Source: CAD feature listing. Evaluate the final solid. Frame: model axes, mm. A direction names the side the tool comes from. Coordinates: 2 decimals unless noted, no trailing zeros. Order: outer loops, then holes, each group sorted by start corner. A loop starts at its lowest first (then second) coordinate and runs counter-clockwise, first axis right, second up.
Autodesk Inventor part; units mm, degrees
ref_plane "YZ Plane" through (0, 0, 0) normal (1, 0, 0) x (0, 1, 0)
ref_plane "XZ Plane" through (0, 0, 0) normal (0, 1, 0) x (-1, 0, 0)
ref_plane "XY Plane" through (0, 0, 0) normal (0, 0, 1) x (1, 0, 0)
sketch "Sketch1" plane through (0, 0, 0) normal (0, 0, 1) x (1, 0, 0)
  line L0 (0, 0) -> (-50.8, 0)
  line L1 (-50.8, 0) -> (-50.8, -12.7)
  line L2 (-50.8, -12.7) -> (-38.1, -12.7)
  line L3 (-12.0663, -25.4) -> (-12.0663, -48.26)
  line L4 (-5, -48.26) -> (-5, -16.764)
  line L5 (-5, -16.764) -> (0, -16.764)
  line L6 (0, -16.764) -> (0, 0)
  line L7 (-12.0663, -48.26) -> (-5, -48.26)
  line L8 (-38.1, -12.7) -> (-38.1, -25.4)
  line L9 (-38.1, -25.4) -> (-12.0663, -25.4)
  dimension "d0" = 50.8
  dimension "d1" = 5
  dimension "d2" = 12.0663
  dimension "d13" = 35.56
  dimension "d15" = 31.496
  dimension "d38" = 12.7
  dimension "d39" = 38.1
revolve "Revolution1" add sketch "Sketch1" angle 360 about axis through (0, -16.764, 0) along (0, 1, 0)
sketch "Sketch5" plane through (0, 0, 0) normal (0, 1, 0) x (1, 0, 0)
  circle A0 centre (0, 0) radius 5
  line L0 (9.815, 0) -> (4.9075, -8.5)
  line L1 (4.9075, -8.5) -> (-4.9075, -8.5)
  line L2 (-4.9075, -8.5) -> (-9.815, 0)
  line L3 (-9.815, 0) -> (-4.9075, 8.5)
  line L4 (-4.9075, 8.5) -> (4.9075, 8.5)
  line L5 (4.9075, 8.5) -> (9.815, 0)
  point P0 (0, 0)
  point P1 (0, 0)
  dimension "d16" = 17
extrude "Extrusion1" cut sketch "Sketch5" against normal blind 12.7 contours A0 | L0 L1 L2 L3 L4 L5
sketch "Sketch7" plane through (0, -12.7, 0) normal (0, -1, 0) x (1, 0, 0)
  circle A0 centre (0, 0) radius 50.8
  line L0 (47.0929, -19.05) -> (85.1929, -19.05)
  line L1 (85.1929, -19.05) -> (85.1929, -31.75)
  line L2 (85.1929, -31.75) -> (39.6557, -31.75)
  circle A1 centre (0, 0) radius 5 construction
  line L3 (0, 0) -> (5, 0) construction
  line L4 (50.8, 0) -> (83.823, 0) construction
  dimension "d23" = 38.1
  dimension "d24" = 12.7
  dimension "d25" = 19.05
extrude "Extrusion3" add sketch "Sketch7" against normal blind 12.7 contours A0 L0 L1 L2
sketch "Sketch8" plane through (39.6557, 0, -31.75) normal (0, 1, 0) x (1, 0, 0)
  line L0 (45.5371, -12.7) -> (45.5371, 0)
  line L1 (45.5371, 0) -> (0, 0)
  line L2 (7.4371, -12.7) -> (45.5371, -12.7)
  line L3 (35.8511, -107.95) -> (35.8511, 44.45)
  line L4 (26.3261, -107.95) -> (26.3261, 44.45)
  line L5 (45.5371, -12.7) -> (23.3121, -12.7)
  line L6 (23.3121, -12.7) -> (23.3121, 0)
  line L7 (23.3121, 0) -> (45.5371, 0)
  line L8 (45.5371, 0) -> (45.5371, -12.7)
  point P0 (-39.6557, -31.75)
  point P1 (23.3121, 0)
  point P2 (23.3121, -12.7)
  dimension "d28" = 22.225
extrude "Extrusion4" add sketch "Sketch8" along normal blind 19.05
sketch "Sketch9" plane through (85.1929, -12.7, -31.75) normal (0, 0, -1) x (-1, 0, 0)
  line L0 (22.225, 12.7) -> (22.225, 31.75)
  line L1 (0, 31.75) -> (22.225, 31.75)
  arc A0 (16.0423, 14.3621) -> (12.8546, 14.3621) centre (14.4485, 18.85) ccw
  line L2 (0, 0) -> (0, 31.75)
  circle A1 centre (14.4485, 18.85) radius 4.953
  point P0 (85.1929, 12.7)
  dimension "d31" = 9.906
extrude "Extrusion5" cut sketch "Sketch9" against normal through all
mirror "Mirror1" about plane through (0, 0, 0) normal (0, 0, 1) of "Extrusion4", "Extrusion5", "Extrusion3"
sketch "Sketch10" plane through (39.6557, -12.7, -31.75) normal (0, -1, 0) x (1, 0, 0)
  arc A0 (7.4371, 12.7) -> (7.4371, 50.8) centre (-39.6557, 31.75) ccw
  line L0 (45.5371, 50.8) -> (7.4371, 50.8)
  line L1 (45.5371, 12.7) -> (7.4371, 12.7)
  arc A1 (7.4371, 12.7) -> (7.4371, 50.8) centre (-39.6557, 31.75) ccw
  line L2 (7.4371, 50.8) -> (45.5371, 50.8)
  line L3 (45.5371, 0) -> (45.5371, 12.7)
  line L4 (45.5371, 50.8) -> (45.5371, 12.7)
  line L5 (45.5371, 12.7) -> (7.4371, 12.7)
extrude "Extrusion6" add sketch "Sketch10" against normal blind 6.35
sketch "Sketch11" plane through (85.1929, -12.7, -31.75) normal (1, 0, 0) x (0, 0, -1)
  line L0 (-63.5, 0) -> (-63.5, 31.75)
  line L1 (-50.8, 31.75) -> (-63.5, 31.75)
  line L2 (-12.7, 31.75) -> (0, 31.75)
  line L3 (0, 0) -> (0, 31.75)
  line L4 (0, 0) -> (-63.5, 0)
  line L5 (-63.5, 31.75) -> (0, 31.75)
  line L6 (0, 31.75) -> (0, 0)
  line L7 (0, 0) -> (-63.5, 0)
  line L8 (-63.5, 0) -> (-63.5, 31.75)
  point P0 (-31.75, 12.7)
  point P1 (-12.7, 31.75)
  point P2 (-50.8, 31.75)
extrude "Extrusion7" add sketch "Sketch11" along normal blind 6.35
sketch "Sketch12" plane through (39.6557, 19.05, -31.75) normal (0, 1, 0) x (1, 0, 0)
  point P0 (-39.6557, -31.75)
sketch "Sketch13" plane through (0, -12.7, 0) normal (0, -1, 0) x (1, 0, 0)
  circle A0 centre (0, 0) radius 5
  line L0 (91.5429, -31.75) -> (91.5429, 31.75)
  circle A1 centre (0, 0) radius 96.8925
  point P0 (0, 0)
extrude "Extrusion8" cut sketch "Sketch13" against normal through all contours A1 L0 picked at (62.6952, 0)
equation "\"d0\" = topPartRadius"
equation "\"d2\" = stemRadius"
equation "\"d15\" = internalHoleDepth"
equation "\"topPartRadius\" = 0.5 * topPartDiameter"
equation "\"totalHeight\" = 35.56"
equation "\"stemRadius\" = 12.06627"
equation "\"stemHeight\" = 22.86"
equation "\"internalHoleDepth\" = 31.496"
equation "\"topPartDiameter\" = 101.6"
properties part number "celestronTripodAdapterBottom" material "PC/ABS Plastic"
1. Draft query along X for faces 1 (the face through (-6.49, -36.99, -10.17)), 2 (the face through (0, -16.764, 0)), 3 (the face through (9, -25.4, 9)). Return one class per face: released by +X, released by -X, zero draft, split by the parting line, or undercut.
Findings:
face 1: split by the parting line
face 2: undercut
face 3: zero draft
2. Ray query, line 1 (Z direction, x = 0, y = -36); line 2 (Y direction, x = 28, z = 1.5); line 3 (X direction, y = -34.5, z = -0.5). Return the intervals inside material, ascending.
Findings:
line 1: z = -12.07 to -5, 5 to 12.07
line 2: y = -25.4 to -12.7
line 3: x = -12.06 to -4.97, 4.97 to 12.06
3. Section query A-A on z = 0. Return loops of the section in (x, y), plus the area to 3 significant figures.
Findings:
outline: (-38.1, -25.4) - (-12.07, -25.4) - (-12.07, -48.26) - (-5, -48.26) - (-5, -16.76) - (5, -16.76) - (5, -48.26) - (12.07, -48.26) - (12.07, -25.4) - (38.1, -25.4) - (38.1, -12.7) - (-38.1, -12.7) - close
area: 1,200 mm2
4. Section query D-D on y = -40. Return loops of the section in (x, z).
Findings:
outline: circle Ø24.13 at (0, 0); hole circle Ø10 at (0, 0)
5. Access query for faces 4 (the face through (30.235, -19.139, 23.183)), 5 (the face through (1.08, -32.29, -4.88)). Directions: +Z, -Z, +X, -X, +Y, -Y. A direction counts if a zero-diameter tool reaches every point of the face in a straight line with its end or side. Return the directions, or none.
Findings:
face 4: +Y, -Y
face 5: -Y
6. Pin query (flat end, axial travel): P1, Ø1, axis at x = -18.5, z = -9, coming from the -Y side; P2, Ø2, axis at x = 18, y = -17, coming from the +Z side; P3, Ø11, axis at x = -2.5, z = -1.5, coming from the -Y side; P4, Ø6, axis at y = -23, z = 9, coming from the -X side. Return the tip coordinate at first contact, or that it passes through.
Findings:
P1: stops at y = -25.4
P2: stops at z = 34.1
P3: stops at y = -48.26
P4: stops at x = -37.62
7. Section query C-C on y = -18. Return loops of the section in (x, z), plus the area to 3 significant figures.
Findings:
outline: circle Ø76.2 at (0, 0); hole circle Ø10 at (0, 0)
area: 4,480 mm2
8. Section query B-B on x = 0. Return loops of the section in (y, z).
Findings:
outline: (-48.26, -12.07) - (-25.4, -12.07) - (-25.4, -38.1) - (-12.7, -38.1) - (-12.7, 38.1) - (-25.4, 38.1) - (-25.4, 12.07) - (-48.26, 12.07) - (-48.26, 5) - (-16.76, 5) - (-16.76, -5) - (-48.26, -5) - close
